```python
from build123d import *

# Parameters (mm, degrees)
F0_W     = 188.5
F0_H     = 4
F0_W_2   = 12
F0_H_2   = 2
F0_W_3   = 238
F2_R     = 22
F2_R_2   = 19
F3_DEPTH = 15
F4_R     = 19
F4_R_2   = 9.5
F5_DEPTH = 20


with BuildPart() as f1:
    # F0 (on Front) → F1 (revolve)
    with BuildSketch(Plane.XZ):
        Polygon((28, 6.5574385243), (28, 0), (29.5, 0), (29.5, 4), (29.5, 26.25), (218, 26.25), (218, 27.75), (28, 27.75), align=None)
        with BuildLine():
            ThreePointArc((21, 6.5574385243), (21.7485631709, 3.3166247904), (22, 0))
            Line((22, 0), (28, 0))
            Line((28, 0), (28, 6.5574385243))
            Line((28, 6.5574385243), (21, 6.5574385243))
        make_face()
        with Locations((123.75, 2)):
            Rectangle(F0_W, F0_H)
        Polygon((456, 4), (456, 0), (458, 0), (458, 22.25), (218, 22.25), (218, 20.25), (456, 20.25), align=None)
        with Locations((212, 21.25)):
            Rectangle(F0_W_2, F0_H_2)
        with Locations((337, 2)):
            Rectangle(F0_W_3, F0_H)
        Polygon((458, 22.25), (458, 0), (464, 0), (464, 8), (464, 20), align=None)
        with BuildLine():
            Line((464, 8), (464, 0))
            Line((464, 0), (474, 0))
            ThreePointArc((474, 0), (474.2514368291, 3.3166247904), (475, 6.5574385243))
            Line((475, 6.5574385243), (475, 8))
            Line((475, 8), (464, 8))
        make_face()
        with BuildLine():
            ThreePointArc((475, 6.5574385243), (474.2514368291, 3.3166247904), (474, 0))
            Line((474, 0), (475, 0))
            Line((475, 0), (475, 6.5574385243))
        make_face()
    revolve(axis=Axis((242.75, 0, 0), (-1, 0, 0)))

    # F2 (on Front) → F3 (join, symmetric)
    with BuildSketch(Plane.XZ):
        Circle(F2_R)
        Circle(F2_R_2, mode=Mode.SUBTRACT)
        with BuildLine():
            ThreePointArc((518, 0), (499.3166247904, 21.7485631709), (475, 6.5574385243))
            Line((475, 6.5574385243), (475, -6.5574385243))
            ThreePointArc((475, -6.5574385243), (499.3166247904, -21.7485631709), (518, 0))
        make_face()
        with Locations((496, 0)):
            Circle(F2_R_2, mode=Mode.SUBTRACT)
        with BuildLine():
            Line((475, -6.5574385243), (475, 6.5574385243))
            ThreePointArc((475, 6.5574385243), (474, 0), (475, -6.5574385243))
        make_face()
    extrude(amount=F3_DEPTH, both=True)

    # F4 (on Front) → F5 (join, symmetric)
    with BuildSketch(Plane.XZ):
        Circle(F4_R)
        Circle(F4_R_2, mode=Mode.SUBTRACT)
        with Locations((496, 0)):
            Circle(F4_R)
        with Locations((496, 0)):
            Circle(F4_R_2, mode=Mode.SUBTRACT)
    extrude(amount=F5_DEPTH, both=True)


solid = f1.part
```
Geometry check sheet. Reference: the model listing, model coordinates, mm. A direction names the side the tool comes from. Give positions to 0.01 mm unless a question says otherwise; leave off trailing zeros. Loops run counter-clockwise (first coordinate to the right, second up) from the corner with the lowest first, then second, coordinate; pieces in that order, holes last. Notation, with made-up numbers: M 7.5,52.25 L 61.5,52.25 A5 ccw 61.5,56.25 Z; hole C 51.5,-27 d5. An arc over 180 degrees is marked long. Write item = value, one per line. Start each with the question number.
1. Section check C-C, the plane x = 198. Enter the section's corners in (y, z).
2. Section check A-A, the plane x = 329. Enter the section's corners in (y, z), plus the area to 3 significant figures.
3. Draft check along Z on faces 4 (the face through (333, 17, 11)), 5 (the face through (-9, 20, -4)), 6 (the face through (469.42, -3.06, 7.39)). Enter one of: +Z half, -Z half, draft (parallel to the pull), parting line (faces both ways), or undercut.
4. Go/stop test with flat-tipped pins: P1, Ø11.5, axis at x = 487.5, z = 4, coming from the +Y side; P2, Ø22, axis at x = 488.5, z = 9.5, coming from the -Y side; P3, Ø2, axis at y = 11, z = -15, coming from the +X side. Record where each tip stops, or that it passes through.
5. Thickness scan on probe 1 along Y at (x, z) = (339, 0.5); probe 2 along X at (y, z) = (0, 13); probe 3 along X at (y, z) = (11, 7). Record the ranges inside material, lowest first.
6. Section check B-B, the plane x = 0. Enter the section's corners in (y, z).
7. Tool access check on faces 1 (the face through (489, -15, 18)), 2 (the face through (500, -20, 9)), 3 (the face through (206, -20, -5)). Record the directions out of +Z, -Z, +X, -X, +Y, -Y that give a thin tool (end or side, any length) a straight path to the whole face; none if there is none.
Values follow:
q1.outline = C 0,0 d55.5; C 0,0 d8; hole C 0,0 d52.5
q2.outline = C 0,0 d44.5; C 0,0 d8; hole C 0,0 d40.5
q2.area = 317 mm^2
q3.face_4 = undercut
q3.face_5 = draft
q3.face_6 = parting line
q4.P1 = 20
q4.P2 = -20
q4.P3 = 512.97
q5.probe_1 = -22.24 to -20.24, -3.97 to 3.97, 20.24 to 22.24
q5.probe_2 = -17.75 to 17.75, 28 to 29.5, 456 to 464, 478.25 to 513.75
q5.probe_3 = -20.86 to -6.42, 6.42 to 20.86, 28 to 29.5, 456 to 464, 475.14 to 489.58, 502.42 to 516.86
q6.outline = M -20,-19 L -15,-19 L -15,-22 L 15,-22 L 15,-19 L 20,-19 L 20,-9.5 L -20,-9.5 Z; M -20,9.5 L 20,9.5 L 20,19 L 15,19 L 15,22 L -15,22 L -15,19 L -20,19 Z
q7.face_1 = -Y
q7.face_2 = +Z, -Z, +X, -Y
q7.face_3 = none
